Could you check a few things on this model? Use its own coordinates, in mm. A direction names the side the tool comes from. Round coordinates to 2 decimals unless told otherwise and drop trailing zeros. Loops run counter-clockwise (first coordinate to the right, second up) from the corner with the lowest first, then second, coordinate; pieces in that order, holes last. Notation, with made-up numbers: M -10.75,85.25 L 0.25,85.25 A11 ccw 0.25,91.25 Z; hole C -31,27 d7. An arc over 180 degrees is marked long. Answer in a Markdown table with one row per item.
Solid Edge part; units mm, degrees
sketch "Sketch1" plane through (0, 0, 0) normal (0, 0, 1) x (1, 0, 0)
  line L0 (90, 0) -> (90, 103)
  line L1 (90, 103) -> (45, 103)
  line L2 (0, 67) -> (45, 103)
  line L3 (0, 0) -> (0, 67)
  line L4 (0, 0) -> (90, 0)
extrude "Protrusion1" add sketch "Sketch1" along normal blind 50
sketch "Sketch2" plane through (90, 51.5, 25) normal (1, 0, 0) x (0, 1, 0)
  line L0 (5.5, 7) -> (5.5, 25)
  line L1 (29.5, 7) -> (5.5, 7)
  line L2 (29.5, 25) -> (29.5, 7)
extrude "Cutout1" cut sketch "Sketch2" against normal up to next material side at (90, 57.05, 41)
sketch "Sketch3" plane through (67.5, 103, 25) normal (0, 1, 0) x (0, 0, -1)
  line L0 (7, -22.5) -> (7, 17.5)
  line L1 (7, 17.5) -> (25, 17.5)
extrude "Cutout2" cut sketch "Sketch3" against normal up to next material side at (70, 103, 17.95)
sketch "Sketch4" plane through (67.5, 103, 25) normal (0, 1, 0) x (1, 0, 0)
  line L0 (-42.5122, 5) -> (-51.8826, 5)
  line L1 (-51.8826, 5) -> (-51.8826, 17)
  line L2 (-51.8826, 17) -> (-42.5122, 17)
  line L3 (-42.5122, 17) -> (-42.5122, 5)
extrude "Cutout3" cut sketch "Sketch4" against normal up to next
sketch "Sketch5" plane through (90, 51.5, 25) normal (1, 0, 0) x (0, 1, 0)
  line L0 (-6.5, 5) -> (-51.5, 5)
  line L1 (-6.5, 25) -> (-6.5, 5)
extrude "Cutout4" cut sketch "Sketch5" against normal up to next material side at (90, 22.5, 30.05)
1) I want a section at D-D, the plane z = 10. Please give me the cut outline in (x, y).
Computed:
| item | result |
|---|---|
| outline | M 0,0 L 15.62,0 L 15.62,79.49 L 0,67 Z; M 24.99,0 L 50,0 L 50,103 L 45,103 L 24.99,86.99 Z |
2) I want a section at C-C, the plane x = 47.5. Please give me the cut outline in (y, z).
Computed:
| item | result |
|---|---|
| outline | M 0,0 L 103,0 L 103,50 L 81,50 L 81,32 L 57,32 L 57,50 L 45,50 L 45,30 L 0,30 Z |
3) I need wall thicknesses on line 1 (Y direction, x = 80, z = 44); line 2 (Z direction, x = 21, y = 51); line 3 (X direction, y = 40.5, z = 15.5). Which ranges of each line are inside material? Lowest first, please.
Computed:
| item | result |
|---|---|
| line 1 | y = 45 to 57, 81 to 103 |
| line 2 | z = 0 to 8, 20 to 50 |
| line 3 | x = 0 to 15.62, 24.99 to 50 |
4) I want a section at A-A, the plane z = 36. Please give me the cut outline in (x, y).
Computed:
| item | result |
|---|---|
| outline | M 0,45 L 90,45 L 90,57 L 0,57 Z; M 17.5,81 L 90,81 L 90,103 L 45,103 Z |
5) Which directions (+Z, -Z, +X, -X, +Y, -Y) give clear straight access to the entire face, cutting with the end or side of a thin tool? Please do faces 5 (the face through (46, 57, 41)), 6 (the face through (15.617, 40, 14)), 7 (the face through (46, 23, 30)), 8 (the face through (50, 52, 9)).
Computed:
| item | result |
|---|---|
| face 5 | +Z, +X, -X |
| face 6 | +Y, -Y |
| face 7 | +Z, +X, -X, -Y |
| face 8 | -Z, +X, +Y, -Y |
6) Will these pins go through, and if not, where does the flat tip stop? P1, Ø8, axis at x = 18, y = 32.5, coming from the +Z side; P2, Ø5.5, axis at x = 47, z = 42, coming from the -Y side; P3, Ø9, axis at y = 35, z = 6.5, coming from the +X side.
Computed:
| item | result |
|---|---|
| P1 | stops at z = 30 |
| P2 | stops at y = 45 |
| P3 | stops at x = 50 |
7) If we mould it in two halves opening along Y, with no side actions, what happens to faces 1 (the face through (90, 62, 30)), 2 (the face through (54, 81, 41)), 3 (the face through (46, 45, 40)), 4 (the face through (46, 69, 32))? For each: released by +Y, released by -Y, zero draft, split by the parting line, or undercut.
Computed:
| item | result |
|---|---|
| face 1 | zero draft |
| face 2 | undercut |
| face 3 | released by -Y |
| face 4 | undercut |
8) I want a section at B-B, the plane y = 52. Please give me the cut outline in (x, z).
Computed:
| item | result |
|---|---|
| outline | M 0,0 L 50,0 L 50,18 L 90,18 L 90,50 L 0,50 Z; hole M 15.62,8 L 24.99,8 L 24.99,20 L 15.62,20 Z |
